from build123d import *

# Parameters (mm, degrees)
ESQUISSE1_R             = 3
SUPPORT_DEPTH           = 0.6
ESQUISSE1_4_R           = 2.25
FIXATION_DEPTH          = 0.9
LANGUETTE_DEPTH         = 2.3
ESQUISSE2_R             = 5
ESQUISSE2_R_2           = 4
SEMELLE_DEPTH           = 0.4
ESQUISSE2_4_R           = 3
BOUTONS_DEPTH           = 3
ESQUISSE2_5_R           = 4
ESQUISSE2_5_R_2         = 3
BORDURE_DEPTH           = 2.2
CHANFREIN_SIZE          = 2
CHANFREIN_SIZE_2        = 1
ESQUISSE3_R             = 2.4
ENL_V_MAT_EXTRU_1_DEPTH = 0.01


with BuildPart() as part:
    # Esquisse1 → Support (new body)
    with BuildSketch(Plane(origin=(0, 0, 0), x_dir=(1, 0, 0), z_dir=(0, 1, 0))):
        with BuildLine():
            Line((12.7, 11.75), (-9.7, 11.75))
            Line((-9.7, 11.75), (-21.676479721, 2.492223081))
            ThreePointArc((-21.676479721, 2.492223081), (-18.361819738, 2.82762366), (-16.6, 0))
            ThreePointArc((-16.6, 0), (-18.361819738, -2.82762366), (-21.676479721, -2.492223081))
            Line((-21.676479721, -2.492223081), (-9.7, -11.75))
            Line((-9.7, -11.75), (12.7, -11.75))
            ThreePointArc((12.7, -11.75), (14.125401288, -9.990303879), (15.308839134, -8.059559428))
            ThreePointArc((15.308839134, -8.059559428), (14.701052578, -8.248227129), (14.512384877, -7.640440572))
            ThreePointArc((14.512384877, -7.640440572), (16.4, 0), (14.512384877, 7.640440572))
            ThreePointArc((14.512384877, 7.640440572), (14.701052578, 8.248227129), (15.308839134, 8.059559428))
            ThreePointArc((15.308839134, 8.059559428), (14.125401288, 9.990303879), (12.7, 11.75))
        make_face()
        with Locations(Location((0, 0, 0), (0, 0, 270))):
            Circle(ESQUISSE1_R, mode=Mode.SUBTRACT)
    extrude(amount=SUPPORT_DEPTH)

    # Esquisse1<4> → Fixation (add)
    with BuildSketch(Plane(origin=(0, 0, 0), x_dir=(1, 0, 0), z_dir=(0, 1, 0))):
        with BuildLine():
            ThreePointArc((-16.6, 0), (-18.361819738, 2.82762366), (-21.676479721, 2.492223081))
            ThreePointArc((-21.676479721, 2.492223081), (-22.9, 0), (-21.676479721, -2.492223081))
            ThreePointArc((-21.676479721, -2.492223081), (-18.361819738, -2.82762366), (-16.6, 0))
        make_face()
        with Locations(Location((-19.75, 0, 0), (0, 0, 270))):
            Circle(ESQUISSE1_4_R, mode=Mode.SUBTRACT)
    extrude(amount=FIXATION_DEPTH)

    # Esquisse1<5> → Languette (add)
    with BuildSketch(Plane(origin=(0, 0, 0), x_dir=(1, 0, 0), z_dir=(0, 1, 0))):
        with BuildLine():
            ThreePointArc((15.308839134, -8.059559428), (17.3, 0), (15.308839134, 8.059559428))
            ThreePointArc((15.308839134, 8.059559428), (14.701052578, 8.248227129), (14.512384877, 7.640440572))
            ThreePointArc((14.512384877, 7.640440572), (16.4, 0), (14.512384877, -7.640440572))
            ThreePointArc((14.512384877, -7.640440572), (14.701052578, -8.248227129), (15.308839134, -8.059559428))
        make_face()
    extrude(amount=LANGUETTE_DEPTH)

    # Esquisse2 → Semelle (add)
    # profile 1 of 4: a face of its own
    with BuildSketch(Plane(origin=(0, 0.6, 0), x_dir=(1, 0, 0), z_dir=(0, 1, 0))):
        with Locations(Location((-6.75, 6.75, 0), (0, 0, 90))):
            Circle(ESQUISSE2_R)
        with Locations(Location((-6.75, 6.75, 0), (0, 0, 270))):
            Circle(ESQUISSE2_R_2, mode=Mode.SUBTRACT)
    # profile 2 of 4: a face of its own
    with BuildSketch(Plane(origin=(0, 0.6, 0), x_dir=(1, 0, 0), z_dir=(0, 1, 0))):
        with Locations(Location((6.75, 6.75, 0), (0, 0, 90))):
            Circle(ESQUISSE2_R)
        with Locations(Location((6.75, 6.75, 0), (0, 0, 270))):
            Circle(ESQUISSE2_R_2, mode=Mode.SUBTRACT)
    # profile 3 of 4: a face of its own
    with BuildSketch(Plane(origin=(0, 0.6, 0), x_dir=(1, 0, 0), z_dir=(0, 1, 0))):
        with Locations(Location((6.75, -6.75, 0), (0, 0, 270))):
            Circle(ESQUISSE2_R)
        with Locations(Location((6.75, -6.75, 0), (0, 0, 270))):
            Circle(ESQUISSE2_R_2, mode=Mode.SUBTRACT)
    # profile 4 of 4: a face of its own
    with BuildSketch(Plane(origin=(0, 0.6, 0), x_dir=(1, 0, 0), z_dir=(0, 1, 0))):
        with Locations(Location((-6.75, -6.75, 0), (0, 0, 270))):
            Circle(ESQUISSE2_R)
        with Locations(Location((-6.75, -6.75, 0), (0, 0, 270))):
            Circle(ESQUISSE2_R_2, mode=Mode.SUBTRACT)
    extrude(amount=SEMELLE_DEPTH)

    # Esquisse2<4> → Boutons (add)
    with BuildSketch(Plane(origin=(0, 0.6, 0), x_dir=(1, 0, 0), z_dir=(0, 1, 0))):
        with Locations(Location((-6.75, 6.75, 0), (0, 0, 270))):
            Circle(ESQUISSE2_4_R)
        with Locations(Location((6.75, 6.75, 0), (0, 0, 270))):
            Circle(ESQUISSE2_4_R)
        with Locations(Location((6.75, -6.75, 0), (0, 0, 270))):
            Circle(ESQUISSE2_4_R)
        with Locations(Location((-6.75, -6.75, 0), (0, 0, 270))):
            Circle(ESQUISSE2_4_R)
    extrude(amount=BOUTONS_DEPTH)

    # Esquisse2<5> → Bordure (add)
    # profile 1 of 4: a face of its own
    with BuildSketch(Plane(origin=(0, 0.6, 0), x_dir=(1, 0, 0), z_dir=(0, 1, 0))):
        with Locations(Location((-6.75, 6.75, 0), (0, 0, 270))):
            Circle(ESQUISSE2_5_R)
        with Locations(Location((-6.75, 6.75, 0), (0, 0, 270))):
            Circle(ESQUISSE2_5_R_2, mode=Mode.SUBTRACT)
    # profile 2 of 4: a face of its own
    with BuildSketch(Plane(origin=(0, 0.6, 0), x_dir=(1, 0, 0), z_dir=(0, 1, 0))):
        with Locations(Location((6.75, 6.75, 0), (0, 0, 270))):
            Circle(ESQUISSE2_5_R)
        with Locations(Location((6.75, 6.75, 0), (0, 0, 270))):
            Circle(ESQUISSE2_5_R_2, mode=Mode.SUBTRACT)
    # profile 3 of 4: a face of its own
    with BuildSketch(Plane(origin=(0, 0.6, 0), x_dir=(1, 0, 0), z_dir=(0, 1, 0))):
        with Locations(Location((-6.75, -6.75, 0), (0, 0, 270))):
            Circle(ESQUISSE2_5_R)
        with Locations(Location((-6.75, -6.75, 0), (0, 0, 270))):
            Circle(ESQUISSE2_5_R_2, mode=Mode.SUBTRACT)
    # profile 4 of 4: a face of its own
    with BuildSketch(Plane(origin=(0, 0.6, 0), x_dir=(1, 0, 0), z_dir=(0, 1, 0))):
        with Locations(Location((6.75, -6.75, 0), (0, 0, 270))):
            Circle(ESQUISSE2_5_R)
        with Locations(Location((6.75, -6.75, 0), (0, 0, 270))):
            Circle(ESQUISSE2_5_R_2, mode=Mode.SUBTRACT)
    extrude(amount=BORDURE_DEPTH)

    # Chanfrein
    # the kernel refuses this chamfer: 2, 1 mm, written as the material it takes off along each edge
    with BuildSketch(Plane(origin=(6.75, 2.8, -6.75), x_dir=(0, 0, 1), z_dir=(-1, 0, 0))) as chanfrein_piece_1_section:
        Polygon((4, -CHANFREIN_SIZE), (4 - CHANFREIN_SIZE_2, 0), (4, 0), align=None)
    chanfrein_piece_1 = revolve(axis=Axis((6.75, 2.8, -6.75), (0, 1, 0)), mode=Mode.PRIVATE)
    chanfrein_piece_1 = split(chanfrein_piece_1, bisect_by=Plane(origin=(6.75, 1, -10.226430856), z_dir=(0, 1, 0)), keep=Keep.TOP, mode=Mode.PRIVATE)
    chanfrein_piece_1 = chanfrein_piece_1 - Plane(origin=(6.75, 1.913215428, -6.75), x_dir=(0, 0, 1), z_dir=(0, -1, 0)) * Cylinder(3, 16, mode=Mode.PRIVATE)
    add(chanfrein_piece_1, mode=Mode.SUBTRACT)
    with BuildSketch(Plane(origin=(6.75, 2.8, 6.75), x_dir=(0, 0, 1), z_dir=(-1, 0, 0))) as chanfrein_piece_2_section:
        Polygon((4, -CHANFREIN_SIZE), (4 - CHANFREIN_SIZE_2, 0), (4, 0), align=None)
    chanfrein_piece_2 = revolve(axis=Axis((6.75, 2.8, 6.75), (0, 1, 0)), mode=Mode.PRIVATE)
    chanfrein_piece_2 = split(chanfrein_piece_2, bisect_by=Plane(origin=(6.75, 1, 3.273569144), z_dir=(0, 1, 0)), keep=Keep.TOP, mode=Mode.PRIVATE)
    chanfrein_piece_2 = chanfrein_piece_2 - Plane(origin=(6.75, 1.913215428, 6.75), x_dir=(0, 0, 1), z_dir=(0, -1, 0)) * Cylinder(3, 16, mode=Mode.PRIVATE)
    add(chanfrein_piece_2, mode=Mode.SUBTRACT)
    with BuildSketch(Plane(origin=(-6.75, 2.8, 6.75), x_dir=(0, 0, 1), z_dir=(-1, 0, 0))) as chanfrein_piece_3_section:
        Polygon((4, -CHANFREIN_SIZE), (4 - CHANFREIN_SIZE_2, 0), (4, 0), align=None)
    chanfrein_piece_3 = revolve(axis=Axis((-6.75, 2.8, 6.75), (0, 1, 0)), mode=Mode.PRIVATE)
    chanfrein_piece_3 = split(chanfrein_piece_3, bisect_by=Plane(origin=(-6.75, 1, 3.273569144), z_dir=(0, 1, 0)), keep=Keep.TOP, mode=Mode.PRIVATE)
    chanfrein_piece_3 = chanfrein_piece_3 - Plane(origin=(-6.75, 1.913215428, 6.75), x_dir=(0, 0, 1), z_dir=(0, -1, 0)) * Cylinder(3, 16, mode=Mode.PRIVATE)
    add(chanfrein_piece_3, mode=Mode.SUBTRACT)
    with BuildSketch(Plane(origin=(-6.75, 2.8, -6.75), x_dir=(0, 0, 1), z_dir=(-1, 0, 0))) as chanfrein_piece_4_section:
        Polygon((4, -CHANFREIN_SIZE), (4 - CHANFREIN_SIZE_2, 0), (4, 0), align=None)
    chanfrein_piece_4 = revolve(axis=Axis((-6.75, 2.8, -6.75), (0, 1, 0)), mode=Mode.PRIVATE)
    chanfrein_piece_4 = split(chanfrein_piece_4, bisect_by=Plane(origin=(-6.75, 1, -10.226430856), z_dir=(0, 1, 0)), keep=Keep.TOP, mode=Mode.PRIVATE)
    chanfrein_piece_4 = chanfrein_piece_4 - Plane(origin=(-6.75, 1.913215428, -6.75), x_dir=(0, 0, 1), z_dir=(0, -1, 0)) * Cylinder(3, 16, mode=Mode.PRIVATE)
    add(chanfrein_piece_4, mode=Mode.SUBTRACT)

    # Esquisse3 → Enlèv. mat.-Extru.1 (cut)
    with BuildSketch(Plane.XZ):
        with Locations(Location((6.75, -6.75, 0), (0, 0, 270))):
            Circle(ESQUISSE3_R)
        with Locations(Location((-6.75, -6.75, 0), (0, 0, 270))):
            Circle(ESQUISSE3_R)
        with Locations(Location((6.75, 6.75, 0), (0, 0, 270))):
            Circle(ESQUISSE3_R)
        with Locations(Location((-6.75, 6.75, 0), (0, 0, 270))):
            Circle(ESQUISSE3_R)
    extrude(amount=-ENL_V_MAT_EXTRU_1_DEPTH, mode=Mode.SUBTRACT)


solid = part.part
Input: part model. Units: mm. Frame: model coordinates. Give positions to 0.01 mm unless a question says otherwise; leave off trailing zeros. Order: outer loops, then holes, each group sorted by start corner. A loop starts at its lowest first (then second) coordinate and runs counter-clockwise, first axis right, second up. Notation, with made-up numbers: (29.25, -1.5) - (65.25, -1.5) arc R10 ccw to (65.25, 11.5) - close; hole circle Ø1 at (24.5, 7.25). An arc over 180 degrees is marked (long way). Answer as a JSON object with one key per item and string values. Group by question number.
Q1. Cut plane B-B, the plane y = 1.6. Output: boundary loops of the cut face in (x, z).
Q2. Line query: probe 1 along X at (y, z) = (0.4, 0); probe 2 along X at (y, z) = (1.05, -6); probe 3 along Y at (x, z) = (7, 7.25). Output: solid intervals per line, ascending.
Q3. First-contact query: pin 1 Ø2.5 at (x, z) = (6, -6) entering from -Y; pin 2 Ø1 at (x, z) = (-2, -2.5) entering from +Y; pin 3 Ø12 at (x, z) = (10.5, 4.5) entering from +Y; pin 4 Ø2.5 at (x, z) = (-19.75, 0) entering from -Y. Flat tips, straight axial feed; report the tip coordinate or a pass-through.
Q4. Cut plane A-A, the plane x = 0. Output: boundary loops of the cut face in (y, z).
Q5. Cut plane C-C, the plane z = 1. Output: boundary loops of the cut face in (x, y).
Results:
{
 "1": {"outline": "circle Ø7.2 at (-6.75, -6.75); circle Ø7.2 at (-6.75, 6.75); circle Ø7.2 at (6.75, -6.75); circle Ø7.2 at (6.75, 6.75); (14.51, -7.64) arc R0.45 ccw to (15.31, -8.06) arc R17.31 ccw to (15.31, 8.06) arc R0.45 ccw to (14.51, 7.64) arc R16.41 cw to start"},
 "2": {"probe 1": "-22.9 to -22, -17.5 to -3, 3 to 17.3", "probe 2": "-10.55 to -2.95, 2.95 to 10.55, 15.26 to 16.23", "probe 3": "0.01 to 3.6"},
 "3": {"pin 1": "y = 0.01", "pin 2": "y = 0.6", "pin 3": "y = 3.6", "pin 4": "through"},
 "4": {"outline": "(0, -11.75) - (0.6, -11.75) - (0.6, -3) - (0, -3) - close; (0, 3) - (0.6, 3) - (0.6, 11.75) - (0, 11.75) - close"},
 "5": {"outline": "(-22.74, 0) - (-21.77, 0) - (-21.77, 0.9) - (-22.74, 0.9) - close; (-17.73, 0) - (-2.83, 0) - (-2.83, 0.6) - (-16.76, 0.6) - (-16.76, 0.9) - (-17.73, 0.9) - close; (2.83, 0) - (17.27, 0) - (17.27, 2.3) - (16.37, 2.3) - (16.37, 0.6) - (2.83, 0.6) - close"}
}
